Verification items for the finished model (mm, model axes). A direction names the side the tool comes from. Round coordinates to 2 decimals unless told otherwise and drop trailing zeros. Order: outer loops, then holes, each group sorted by start corner. A loop starts at its lowest first (then second) coordinate and runs counter-clockwise, first axis right, second up. Notation, with made-up numbers: M -1,20 L 11,20 A26 ccw 11,35 Z; hole C -24,-15 d4. An arc over 180 degrees is marked long. Use one line per item in the form item = value. Start each with the question number.
Item 1: Tool access check on faces 4 (the flat face through (5, -28, 4)), 5 (the flat face through (7, -20, 7)), 6 (the cylindrical face through (-0.07, 3.077, 10.012)). Record the directions out of +Z, -Z, +X, -X, +Y, -Y that give a thin tool (end or side, any length) a straight path to the whole face; none if there is none.
Item 2: Thickness scan on probe 1 along Z at (x, y) = (-4.5, 23.5); probe 2 along X at (y, z) = (-24, 8.75); probe 3 along Y at (x, z) = (0, 12.6). Record the ranges inside material, lowest first. Write a range as [from, to].
Item 3: Release check for a two-part mould opening along X. For faces 1 (the cylindrical face through (-5.986, 2.81, 2.594)), 2 (the flat face through (-5, -28, 4)), 3 (the cylindrical face through (-0.2, 37.92, 12.48)) record: +X half, -X half, draft (parallel to the pull), parting line (faces both ways), or undercut.
Item 4: Go/stop test with flat-tipped pins: pin 1 Ø4.5 at (y, z) = (-18, 4) entering from +X; pin 2 Ø10 at (x, y) = (-4, -32.5) entering from -Z; pin 3 Ø3 at (x, y) = (-1, -47) entering from +Z. Record where each tip stops, or that it passes through.
Item 5: Cross-section at A-A on y = 22. Enter the section's corners in (x, z).
Item 6: Cross-section at D-D on y = -48.5. Enter the section's corners in (x, z), then the cut area to 3 significant figures.
Item 7: Cross-section at C-C on z = 12.25. Enter the section's corners in (x, y).
Item 8: Cross-section at B-B on x = 0. Enter the section's corners in (y, z), then the cut area to 3 significant figures.
from build123d import *

# Parameters (mm, degrees)
SKETCH1_R               = 5
BOSS_EXTRUDE1_DEPTH     = 14
CUT_EXTRUDE1_DEPTH      = 14
CUT_EXTRUDE1_DEPTH_BACK = 21
CUT_EXTRUDE2_DEPTH      = 26
CUT_EXTRUDE2_DEPTH_BACK = 28
CUT_EXTRUDE3_DEPTH      = 5
CUT_EXTRUDE3_DEPTH_BACK = 5
CUT_EXTRUDE4_START      = -1
CUT_EXTRUDE4_DEPTH      = 1
CUT_EXTRUDE6_START      = -7
CUT_EXTRUDE6_DEPTH      = 1
SKETCH8_R               = 1
CUT_EXTRUDE8_DEPTH      = 15
FILLET2_RADIUS          = 2.5
FILLET2_LENGTH          = 15
FILLET3_RADIUS          = 2.5
FILLET3_LENGTH          = 15
FILLET4_R               = 3
FILLET5_R               = 2
CUT_EXTRUDE9_DEPTH      = 95.601560752
CUT_EXTRUDE9_DEPTH_BACK = 22
CUT_EXTRUDE10_DEPTH     = 19


with BuildPart() as part:
    # Sketch1 → Boss-Extrude1 (new body)
    with BuildSketch(Plane.XY):
        with BuildLine():
            Line((7, 27.728093549), (7, -70.844330052))
            ThreePointArc((7, -70.844330052), (9.983048869, -72.249040285), (12.694763676, -74.124778593))
            ThreePointArc((12.694763676, -74.124778593), (13.290040181, -74.462261791), (13.964240044, -74.579324047))
            Line((13.964240044, -74.579324047), (20, -74.579324047))
            Line((20, -74.579324047), (20, -89.579324047))
            Line((20, -89.579324047), (15, -89.579324047))
            ThreePointArc((15, -89.579324047), (0, -74.579324047), (-15, -89.579324047))
            Line((-15, -89.579324047), (-20, -89.579324047))
            Line((-20, -89.579324047), (-20, -74.579324047))
            Line((-20, -74.579324047), (-13.964240044, -74.579324047))
            ThreePointArc((-13.964240044, -74.579324047), (-13.290040181, -74.462261791), (-12.694763676, -74.124778593))
            ThreePointArc((-12.694763676, -74.124778593), (-9.983048869, -72.249040285), (-7, -70.844330052))
            Line((-7, -70.844330052), (-7, 27.728093549))
            ThreePointArc((-7, 27.728093549), (0, 37.920675953), (7, 27.728093549))
        make_face()
        with Locations((0, 30.420675953)):
            Circle(SKETCH1_R, mode=Mode.SUBTRACT)
    extrude(amount=BOSS_EXTRUDE1_DEPTH)

    # Sketch2 → Cut-Extrude1 (cut, two sides: drawn at the far end of the back side and taken through both)
    with BuildSketch(Plane(origin=(7, 0, 0), x_dir=(0, 0, -1), z_dir=(1, 0, 0)).offset(-CUT_EXTRUDE1_DEPTH_BACK)):
        with BuildLine():
            Line((-11, 19.155669948), (-11, 94.026923789))
            Line((-11, 94.026923789), (-3, 94.026923789))
            Line((-3, 94.026923789), (-3, 19.155669948))
            ThreePointArc((-3, 19.155669948), (-7, 15.155669948), (-11, 19.155669948))
        make_face()
    extrude(amount=CUT_EXTRUDE1_DEPTH + CUT_EXTRUDE1_DEPTH_BACK, mode=Mode.SUBTRACT)

    # Sketch3 → Cut-Extrude2 (cut, two sides: drawn at the far end of the back side and taken through both)
    with BuildSketch(Plane.ZY.offset(7).offset(-CUT_EXTRUDE2_DEPTH_BACK)):
        with BuildLine():
            Line((3.5, -7.579324047), (3.5, -89.579324047))
            Line((3.5, -89.579324047), (0, -89.579324047))
            Line((0, -89.579324047), (0, 12.613496459))
            ThreePointArc((0, 12.613496459), (2.618525015, 2.667626719), (3.5, -7.579324047))
        make_face()
        with BuildLine():
            Line((10.5, -7.579324047), (10.5, -89.579324047))
            Line((10.5, -89.579324047), (14, -89.579324047))
            Line((14, -89.579324047), (14, 12.613496459))
            ThreePointArc((14, 12.613496459), (11.381474985, 2.667626719), (10.5, -7.579324047))
        make_face()
    extrude(amount=CUT_EXTRUDE2_DEPTH + CUT_EXTRUDE2_DEPTH_BACK, mode=Mode.SUBTRACT)

    # Sketch4 → Cut-Extrude3 (cut, two sides: drawn at the far end of the back side and taken through both)
    with BuildSketch(Plane(origin=(0, 0, 0), x_dir=(0, 0, -1), z_dir=(1, 0, 0)).offset(-CUT_EXTRUDE3_DEPTH_BACK)):
        with BuildLine():
            Line((-5.4, -7.457377961), (-5.4, -65.313507329))
            ThreePointArc((-5.4, -65.313507329), (-4.911756575, -68.237545632), (-3.5, -70.844330052))
            Line((-3.5, -70.844330052), (19.637557059, -70.844330052))
            Line((19.637557059, -70.844330052), (19.637557059, 12.613496459))
            Line((19.637557059, 12.613496459), (0, 12.613496459))
            ThreePointArc((0, 12.613496459), (-4.026415832, 2.934926884), (-5.4, -7.457377961))
        make_face()
        with BuildLine():
            Line((-8.6, -7.457377961), (-8.6, -65.313507329))
            ThreePointArc((-8.6, -65.313507329), (-9.088243425, -68.237545632), (-10.5, -70.844330052))
            Line((-10.5, -70.844330052), (-24.530573049, -70.844330052))
            Line((-24.530573049, -70.844330052), (-24.530573049, 12.613496459))
            Line((-24.530573049, 12.613496459), (-14, 12.613496459))
            ThreePointArc((-14, 12.613496459), (-9.973584168, 2.934926884), (-8.6, -7.457377961))
        make_face()
    extrude(amount=CUT_EXTRUDE3_DEPTH + CUT_EXTRUDE3_DEPTH_BACK, mode=Mode.SUBTRACT)

    # Sketch5 → Cut-Extrude4 (cut)
    with BuildSketch(Plane.XY.offset(10.5).offset(CUT_EXTRUDE4_START)):
        with BuildLine():
            Line((-16, -89.579324047), (-20, -89.579324047))
            Line((-20, -89.579324047), (-20, -74.579324047))
            Line((-20, -74.579324047), (-13.964240044, -74.579324047))
            ThreePointArc((-13.964240044, -74.579324047), (-13.290040181, -74.462261791), (-12.694763676, -74.124778593))
            ThreePointArc((-12.694763676, -74.124778593), (0, -69.579324047), (12.694763676, -74.124778593))
            ThreePointArc((12.694763676, -74.124778593), (13.290040181, -74.462261791), (13.964240044, -74.579324047))
            Line((13.964240044, -74.579324047), (20, -74.579324047))
            Line((20, -74.579324047), (20, -89.579324047))
            Line((20, -89.579324047), (16, -89.579324047))
            ThreePointArc((16, -89.579324047), (0, -73.579324047), (-16, -89.579324047))
        make_face()
    extrude(amount=CUT_EXTRUDE4_DEPTH, mode=Mode.SUBTRACT)

    # Sketch5<3> → Cut-Extrude6 (cut)
    with BuildSketch(Plane.XY.offset(10.5).offset(CUT_EXTRUDE6_START)):
        with BuildLine():
            Line((-16, -89.579324047), (-20, -89.579324047))
            Line((-20, -89.579324047), (-20, -74.579324047))
            Line((-20, -74.579324047), (-13.964240044, -74.579324047))
            ThreePointArc((-13.964240044, -74.579324047), (-13.290040181, -74.462261791), (-12.694763676, -74.124778593))
            ThreePointArc((-12.694763676, -74.124778593), (0, -69.579324047), (12.694763676, -74.124778593))
            ThreePointArc((12.694763676, -74.124778593), (13.290040181, -74.462261791), (13.964240044, -74.579324047))
            Line((13.964240044, -74.579324047), (20, -74.579324047))
            Line((20, -74.579324047), (20, -89.579324047))
            Line((20, -89.579324047), (16, -89.579324047))
            ThreePointArc((16, -89.579324047), (0, -73.579324047), (-16, -89.579324047))
        make_face()
    extrude(amount=CUT_EXTRUDE6_DEPTH, mode=Mode.SUBTRACT)

    # Sketch8 → Cut-Extrude8 (cut)
    with BuildSketch(Plane(origin=(0, -74.579324047, 0), x_dir=(1, 0, 0), z_dir=(0, 1, 0))):
        with Locations(Location((17, -7, 0), (0, 0, 270))):
            Circle(SKETCH8_R)
        with Locations(Location((-17, -7, 0), (0, 0, 270))):
            Circle(SKETCH8_R)
    extrude(amount=-CUT_EXTRUDE8_DEPTH, mode=Mode.SUBTRACT)

    # Fillet2: full round fillet: the end face becomes a half cylinder, R = half its width
    fillet2_face = Plane((-20, -82.079324047, 7), x_dir=(0, 1, 0), z_dir=(-1, 0, 0))  # on the end face: x along it, z out of the body
    fillet2_slab = fillet2_face.offset(-FILLET2_RADIUS / 2) * Box(FILLET2_LENGTH, 2 * FILLET2_RADIUS, FILLET2_RADIUS, mode=Mode.PRIVATE)  # the body's end, R deep
    fillet2_round = Plane((-17.5, -82.079324047, 7), x_dir=(-1, 0, 0), z_dir=(0, 1, 0)) * Cylinder(FILLET2_RADIUS, FILLET2_LENGTH, mode=Mode.PRIVATE)  # its axis R under the face
    add(fillet2_slab - fillet2_round, mode=Mode.SUBTRACT)

    # Fillet3: full round fillet: the end face becomes a half cylinder, R = half its width
    fillet3_face = Plane((20, -82.079324047, 7), x_dir=(0, -1, 0), z_dir=(1, 0, 0))  # on the end face: x along it, z out of the body
    fillet3_slab = fillet3_face.offset(-FILLET3_RADIUS / 2) * Box(FILLET3_LENGTH, 2 * FILLET3_RADIUS, FILLET3_RADIUS, mode=Mode.PRIVATE)  # the body's end, R deep
    fillet3_round = Plane((17.5, -82.079324047, 7), x_dir=(1, 0, 0), z_dir=(0, -1, 0)) * Cylinder(FILLET3_RADIUS, FILLET3_LENGTH, mode=Mode.PRIVATE)  # its axis R under the face
    add(fillet3_slab - fillet3_round, mode=Mode.SUBTRACT)

    # Fillet4
    fillet4_edges = [part.edges().sort_by_distance(p)[0] for p in [
        (-7, -70.844330052, 7),
        (7, -70.844330052, 7),
    ]]
    fillet(fillet4_edges, radius=FILLET4_R)

    # Fillet5
    fillet5_edges = [part.edges().sort_by_distance(p)[0] for p in [
        (-7, 27.728093549, 12.5),
        (7, 27.728093549, 12.5),
        (-7, 27.728093549, 1.5),
        (7, 27.728093549, 1.5),
    ]]
    fillet(fillet5_edges, radius=FILLET5_R)

    # Sketch10 → Cut-Extrude9 (cut, two sides: drawn at the far end of the back side and taken through both)
    with BuildSketch(Plane(origin=(7, 0, 0), x_dir=(0, 0, -1), z_dir=(1, 0, 0)).offset(-CUT_EXTRUDE9_DEPTH_BACK)):
        Polygon((-3.5, -55.844330052), (-4.5, -68.86700887), (-4.5, -70.844330052), (-3.5, -70.844330052), align=None)
    extrude(amount=CUT_EXTRUDE9_DEPTH + CUT_EXTRUDE9_DEPTH_BACK, mode=Mode.SUBTRACT)

    # Sketch11 → Cut-Extrude10 (cut)
    with BuildSketch(Plane(origin=(7, 0, 0), x_dir=(0, 0, -1), z_dir=(1, 0, 0))):
        Polygon((-9.5, -70.844330052), (-10.5, -70.844330052), (-10.5, -55.844330052), (-9.5, -68.86700887), align=None)
    extrude(amount=-CUT_EXTRUDE10_DEPTH, mode=Mode.SUBTRACT)


solid = part.part
Output values:
q1.face_4 = -Z
q1.face_5 = +Z, -Z, +X
q1.face_6 = +Z
q2.probe_1 = [0, 3], [11, 14]
q2.probe_2 = [-7, -5], [5, 7]
q2.probe_3 = [9.98, 25.42], [35.42, 37.92]
q3.face_1 = draft
q3.face_2 = undercut
q3.face_3 = parting line
q4.pin_1 = 7
q4.pin_2 = 3.5
q4.pin_3 = 8.6
q5.outline = M -7,0 L 7,0 L 7,3 L -7,3 Z; M -7,11 L 7,11 L 7,14 L -7,14 Z
q6.outline = M -7,3.5 L -5,3.5 L -5,5.4 L 5,5.4 L 5,3.5 L 7,3.5 L 7,10.5 L 5,10.5 L 5,8.6 L -5,8.6 L -5,10.5 L -7,10.5 Z
q6.area = 60.0 mm2
q7.outline = M -7.11,28.02 A2 cw -7,27.38 L -7,6.81 L -5,6.81 L -5,9.24 L 5,9.24 L 5,6.81 L 7,6.81 L 7,27.38 A2 cw 7.11,28.02 A7.5 ccw long Z; hole C 0,30.42 d10
q8.outline = M -74.58,3.5 L -73.58,3.5 L -73.58,4.5 L -69.24,4.5 A9 cw -65.31,5.4 L -7.46,5.4 A40 cw 12.61,0 L 25.42,0 L 25.42,3 L 19.16,3 A4 cw 19.16,11 L 25.42,11 L 25.42,14 L 12.61,14 A40 cw -7.46,8.6 L -65.31,8.6 A9 cw -69.24,9.5 L -73.58,9.5 L -73.58,10.5 L -74.58,10.5 Z; M 35.42,0 L 37.92,0 L 37.92,3 L 35.42,3 Z; M 35.42,11 L 37.92,11 L 37.92,14 L 35.42,14 Z
q8.area = 482 mm2
